The listing builds one solid part. Answer for the finished solid, in the listing's coordinates (mm). Give positions to 0.01 mm unless a question says otherwise; leave off trailing zeros. Write each loop counter-clockwise with the first axis right and the second up, starting at its lowest first coordinate (ties: lowest second). Pieces come first, ordered by that corner, then holes. Notation, with made-up numbers: M 77,-24.75 L 87,-24.75 A29 cw 87,7.25 Z; hole C 49.25,45.25 d11. An arc over 180 degrees is marked long. Answer as a JSON object with one key per item and string values.
```python
from build123d import *

# Parameters (mm, degrees)
SHELL1_T            = -2
SKETCH3_W           = 10
SKETCH3_H           = 30
FILLET1_R           = 1
SKETCH2_R           = 45
BOSS_EXTRUDE2_DEPTH = 2


with BuildPart() as part:
    # Sketch1 → Revolve1 (revolve)
    with BuildSketch(Plane.XY):
        with BuildLine():
            Line((0, 45), (0, 0))
            Line((0, 0), (45, 0))
            ThreePointArc((45, 0), (31.819805153, 31.819805153), (0, 45))
        make_face()
    revolve(axis=Axis((0, 45, 0), (0, -1, 0)))

    # Shell1
    shell1_openings = [part.faces().sort_by_distance(p)[0] for p in [
        (0, 0, 45),
    ]]
    offset(amount=SHELL1_T, openings=shell1_openings, kind=Kind.INTERSECTION)



with BuildPart() as body_2:
    # Sketch3 → Revolve2 (revolve)
    with BuildSketch(Plane.XY):
        with Locations((-5, 15)):
            Rectangle(SKETCH3_W, SKETCH3_H)
    revolve(axis=Axis((0, 30, 0), (0, -1, 0)))

    # Fillet1
    fillet1_edges = [body_2.edges().sort_by_distance(p)[0] for p in [
        (10, 30, 0),
    ]]
    fillet(fillet1_edges, radius=FILLET1_R)


with BuildPart() as part_1:
    add(part.part)

    add(body_2.part)  # Boss-Extrude2 merges body 2
    # Sketch2 → Boss-Extrude2 (add)
    with BuildSketch(Plane(origin=(0, 0, 0), x_dir=(1, 0, 0), z_dir=(0, 1, 0))):
        Circle(SKETCH2_R)
    extrude(amount=BOSS_EXTRUDE2_DEPTH)


solid = part_1.part
```
1. The mould has two halves that part along X. Classify faces 1 (the flat face through (1, 0, 1)), 2 (the cylindrical face through (2.17, 15.69, 9.76)), 3 (the cylindrical face through (20.765, 0.986, 39.923)), 4 (the flat face through (-0.6, 2, -10.15)): released by +X, released by -X, zero draft, split by the parting line, or undercut.
Verdict:
{"face 1": "zero draft", "face 2": "undercut", "face 3": "split by the parting line", "face 4": "undercut"}
2. Flat-ended cylindrical pins translate along their axes: pin 1 (8 mm diameter, centred on y = 21, z = -34, fed in from -X); pin 2 (5 mm diameter, centred on x = -5, z = 34, fed in from -Y); pin 3 (10 mm diameter, centred on x = -12.5, y = 15.5, fed in from -Z); pin 4 (1.5 mm diameter, centred on x = 20.5, y = 25, fed in from +Z). Find the tip coordinate at first contact, or state that the pin passes through.
Verdict:
{"pin 1": "stops at x = -27.05", "pin 2": "stops at y = 0", "pin 3": "stops at z = -42.46", "pin 4": "stops at z = 32.06"}
3. A cutting plane is placed at C-C, the plane y = 8. Give the vertices of the cut face in (x, z), plus the area to 3 significant figures.
Verdict:
{"outline": "C 0,0 d88.57; C 0,0 d20; hole C 0,0 d84.5", "area": "867 mm2"}
4. Consider line 1 along Z through (x, y) = (-2.5, 11); line 2 along Y through (x, z) = (11.5, 30); line 3 along Z through (x, y) = (24.5, 31). Determine where each line is inside the solid, lowest interval first.
Verdict:
{"line 1": "z = -43.56 to -41.49, -9.68 to 9.68, 41.49 to 43.56", "line 2": "y = 0 to 2, 28.58 to 31.51", "line 3": "z = -21.53 to -16.96, 16.96 to 21.53"}
